Verification items for the finished model (mm, model axes). Face numbers are marked on the shaded views. A direction names the side the tool comes from. Give positions to 0.01 mm unless a question says otherwise; leave off trailing zeros. Order: outer loops, then holes, each group sorted by start corner. A loop starts at its lowest first (then second) coordinate and runs counter-clockwise, first axis right, second up. Notation, with made-up numbers: M 73.25,-19 L 101.25,-19 A23 ccw 101.25,14 Z; hole C -5,48.5 d10. An arc over 180 degrees is marked long. Answer as a JSON object with one key per item and string values.
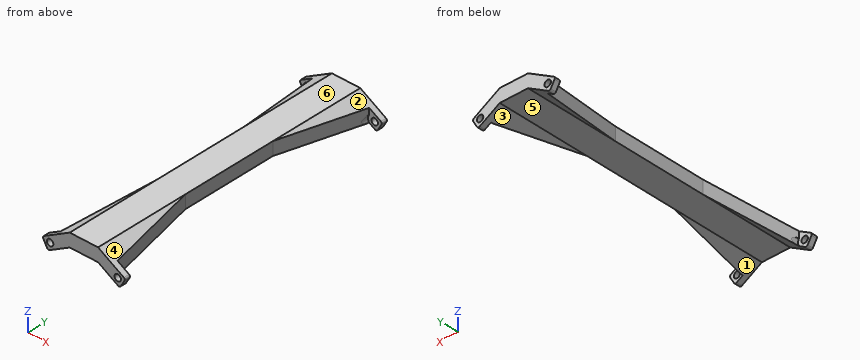
```python
from build123d import *

# Parameters (mm, degrees)
SKETCH2_W            = 15
SKETCH2_H            = 150
BOSS_EXTRUDE1_DEPTH  = 3.5
BOSS_EXTRUDE2_DEPTH  = 150
CUT_EXTRUDE1_DEPTH   = 80.340414561
CUT_EXTRUDE2_REACH   = 150.982
SKETCH6_R            = 1.7
FILLET2_R            = 1
CUT_EXTRUDE3_REACH   = 150.982
SKETCH7_R            = 3.5
FILLET2_OF_MIRROR1_R = 1


with BuildPart() as part:
    # Sketch2 → Boss-Extrude1 (new, symmetric)
    with BuildSketch(Plane.XY):
        Rectangle(SKETCH2_W, SKETCH2_H)
    extrude(amount=BOSS_EXTRUDE1_DEPTH, both=True)

    # Sketch3 → Boss-Extrude2 (add)
    with BuildSketch(Plane.XZ.offset(75)):
        Polygon((-7.5, 3.5), (-22.005925513, -4.875), (-18.9748366, -10.125), (-7.5, -3.5), align=None)
        Polygon((7.5, 3.5), (22.005925513, -4.875), (18.9748366, -10.125), (7.5, -3.5), align=None)
    extrude(amount=-BOSS_EXTRUDE2_DEPTH)

    # Sketch5 → Cut-Extrude1 (cut, through all)
    with BuildSketch(Plane.XY.offset(3.5)):
        Polygon((-7.5, 25), (-7.5, -25), (-15.005925513, -72), (-22.005925513, -72), (-22.005925513, 72), (-15.005925513, 72), align=None)
        Polygon((22.005925513, -72), (15.005925513, -72), (7.5, -25), (7.5, 25), (15.005925513, 72), (22.005925513, 72), align=None)
    extrude(amount=-CUT_EXTRUDE1_DEPTH, mode=Mode.SUBTRACT)

    # Sketch6 → Cut-Extrude2 (cut, up to next)
    with BuildSketch(Plane(origin=(0, -72, 0), x_dir=(1, 0, 0), z_dir=(0, 1, 0)), mode=Mode.PRIVATE) as cut_extrude2_sk1:
        with Locations(Location((17.892304845, 6, 0), (0, 0, 270))):
            Circle(SKETCH6_R)
    cut_extrude2_tool1 = extrude(cut_extrude2_sk1.sketch, amount=-CUT_EXTRUDE2_REACH, mode=Mode.PRIVATE) & part.part
    # Sketch6 → Cut-Extrude2 (cut, up to next)
    with BuildSketch(Plane(origin=(0, -72, 0), x_dir=(1, 0, 0), z_dir=(0, 1, 0)), mode=Mode.PRIVATE) as cut_extrude2_sk2:
        with Locations(Location((-17.892304845, 6, 0), (0, 0, 270))):
            Circle(SKETCH6_R)
    cut_extrude2_tool2 = extrude(cut_extrude2_sk2.sketch, amount=-CUT_EXTRUDE2_REACH, mode=Mode.PRIVATE) & part.part
    cut_extrude2_1 = cut_extrude2_tool1.solids().sort_by_distance((17.892305, -72, -6))[0]
    add(cut_extrude2_1, mode=Mode.SUBTRACT)
    cut_extrude2_2 = cut_extrude2_tool2.solids().sort_by_distance((-17.892305, -72, -6))[0]
    add(cut_extrude2_2, mode=Mode.SUBTRACT)
    cut_extrude2 = cut_extrude2_1 + cut_extrude2_2  # Cut-Extrude2 as one shape, for the pattern or mirror that repeats it

    # Fillet2
    fillet2_edges = [part.edges().sort_by_distance(p)[0] for p in [
        (18.9748366, -73.5, -10.125),
        (22.005925513, -73.5, -4.875),
        (-22.005925513, -73.5, -4.875),
        (-18.9748366, -73.5, -10.125),
    ]]
    fillet(fillet2_edges, radius=FILLET2_R)

    # Sketch7 → Cut-Extrude3 (cut, up to next)
    with BuildSketch(Plane(origin=(0, -72, 0), x_dir=(1, 0, 0), z_dir=(0, 1, 0)), mode=Mode.PRIVATE) as cut_extrude3_sk1:
        with Locations((-17.892304845, 6)):
            Circle(SKETCH7_R)
    cut_extrude3_tool1 = extrude(cut_extrude3_sk1.sketch, amount=CUT_EXTRUDE3_REACH, mode=Mode.PRIVATE) & part.part
    # Sketch7 → Cut-Extrude3 (cut, up to next)
    with BuildSketch(Plane(origin=(0, -72, 0), x_dir=(1, 0, 0), z_dir=(0, 1, 0)), mode=Mode.PRIVATE) as cut_extrude3_sk2:
        with Locations((17.892304845, 6)):
            Circle(SKETCH7_R)
    cut_extrude3_tool2 = extrude(cut_extrude3_sk2.sketch, amount=CUT_EXTRUDE3_REACH, mode=Mode.PRIVATE) & part.part
    cut_extrude3_1 = cut_extrude3_tool1.solids().sort_by_distance((-17.892305, -72, -6))[0]
    add(cut_extrude3_1, mode=Mode.SUBTRACT)
    cut_extrude3_2 = cut_extrude3_tool2.solids().sort_by_distance((17.892305, -72, -6))[0]
    add(cut_extrude3_2, mode=Mode.SUBTRACT)
    cut_extrude3 = cut_extrude3_1 + cut_extrude3_2  # Cut-Extrude3 as one shape, for the pattern or mirror that repeats it

    # Mirror1: Cut-Extrude2, Cut-Extrude3 across plane
    add(cut_extrude2.mirror(Plane.ZX), mode=Mode.SUBTRACT)
    add(cut_extrude3.mirror(Plane.ZX), mode=Mode.SUBTRACT)

    # Fillet2 of Mirror1
    fillet2_of_mirror1_edges = [part.edges().sort_by_distance(p)[0] for p in [
        (18.9748366, 73.5, -10.125),
        (22.005925513, 73.5, -4.875),
        (-22.005925513, 73.5, -4.875),
        (-18.9748366, 73.5, -10.125),
    ]]
    fillet(fillet2_of_mirror1_edges, radius=FILLET2_OF_MIRROR1_R)


solid = part.part
```
Q1. Release check for a two-part mould opening along X. For the marked faces 3, 4, 5 and 6 record: +X half, -X half, draft (parallel to the pull), parting line (faces both ways), or undercut.
Resolved:
{"face 3": "undercut", "face 4": "+X half", "face 5": "undercut", "face 6": "draft"}
Q2. Section check B-B on y = -38. Record the cut outline in (x, z).
Resolved:
{"outline": "M -9.58,-4.7 L -7.5,-3.5 L 7.5,-3.5 L 9.58,-4.7 L 9.58,2.3 L 7.5,3.5 L -7.5,3.5 L -9.58,2.3 Z"}
Q3. Section check A-A on x = 10.5. Record the cut outline in (y, z), then the cut area to 3 significant figures.
Resolved:
{"outline": "M -75,-5.23 L -43.79,-5.23 L -43.79,1.77 L -75,1.77 Z; M 43.79,-5.23 L 75,-5.23 L 75,1.77 L 43.79,1.77 Z", "area": "437 mm²"}
Q4. Tool access check on the marked faces 1 and 2. Record the directions out of +Z, -Z, +X, -X, +Y, -Y that give a thin tool (end or side, any length) a straight path to the whole face; none if there is none.
Resolved:
{"face 1": "-Z, +Y, -Y", "face 2": "+Z, +X, +Y, -Y"}
Q5. Gauge pin test, flat ends, axial feed: pin 1 Ø5.5 at (x, z) = (17.89, -6) entering from +Y; pin 2 Ø4 at (y, z) = (8.5, -6.5) entering from +X; pin 3 Ø12 at (x, y) = (0.5, -49.5) entering from -Z; pin 4 Ø3.5 at (y, z) = (4.5, 0.5) entering from +X. Record the tip position at first contact, or that the pin passes through.
Resolved:
{"pin 1": "stops at y = 75", "pin 2": "passes through", "pin 3": "stops at z = -3.5", "pin 4": "stops at x = 7.5"}
Q6. Section check D-D on y = -5. Record the cut outline in (x, z).
Resolved:
{"outline": "M -7.5,-3.5 L 7.5,-3.5 L 7.5,3.5 L -7.5,3.5 Z"}
Q7. Material ranges on L1, parallel to X at y = -72.95, z = -6; L2, parallel to Y at x = 15, z = -5; L3, parallel to X at y = 20, z = -1.5, recorded low to high.
Resolved:
{"L1": "x = -21.36 to -19.59, -16.19 to -11.83, 11.83 to 16.19, 19.59 to 21.36", "L2": "y = -75 to -72, 72 to 75", "L3": "x = -7.5 to 7.5"}
Q8. Section check C-C on y = 58. Record the cut outline in (x, z).
Resolved:
{"outline": "M -12.77,-6.54 L -7.5,-3.5 L 7.5,-3.5 L 12.77,-6.54 L 12.77,0.46 L 7.5,3.5 L -7.5,3.5 L -12.77,0.46 Z"}
